For this review, take the finished solid that the model builds, in its own axes (mm). Face numbers are marked on the shaded views. A direction names the side the tool comes from. Give positions to 0.01 mm unless a question says otherwise; leave off trailing zeros. Order: outer loops, then holes, each group sorted by start corner. A loop starts at its lowest first (then second) coordinate and runs counter-clockwise, first axis right, second up.
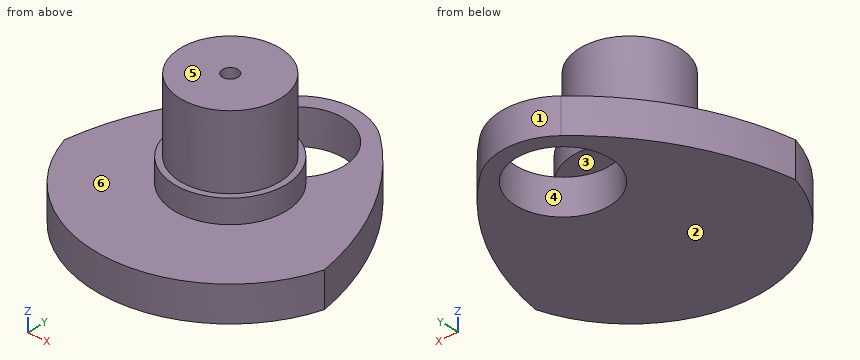
from build123d import *

# Parameters (mm, degrees)
SKETCH3_R           = 17
BOSS_EXTRUDE2_DEPTH = 25
SKETCH4_R           = 19
BOSS_EXTRUDE3_DEPTH = 8
BOSS_EXTRUDE4_DEPTH = 12
SKETCH9_R           = 16
CUT_EXTRUDE1_DEPTH  = 12
SKETCH10_R          = 2.65
CUT_EXTRUDE2_DEPTH  = 15


with BuildPart() as part:
    # Sketch3 → Boss-Extrude2 (new body)
    with BuildSketch(Plane.XY):
        Circle(SKETCH3_R)
    extrude(amount=BOSS_EXTRUDE2_DEPTH)

    # Sketch4 → Boss-Extrude3 (add)
    with BuildSketch(Plane.XY):
        Circle(SKETCH4_R)
    extrude(amount=-BOSS_EXTRUDE3_DEPTH)

    # Sketch5 → Boss-Extrude4 (add)
    with BuildSketch(Plane(origin=(0, 0, -8), x_dir=(-1, 0, 0), z_dir=(0, 0, -1))):
        with BuildLine():
            ThreePointArc((-44, -13.416407865), (0, -46), (44, -13.416407865))
            ThreePointArc((44, -13.416407865), (33.683444249, 16.469257624), (13.668094758, 40.943123461))
            ThreePointArc((13.668094758, 40.943123461), (0, 46), (-13.668094758, 40.943123461))
            ThreePointArc((-13.668094758, 40.943123461), (-33.683444249, 16.469257624), (-44, -13.416407865))
        make_face()
    extrude(amount=BOSS_EXTRUDE4_DEPTH)

    # Sketch9 → Cut-Extrude1 (cut)
    with BuildSketch(Plane(origin=(0, 0, -20), x_dir=(-1, 0, 0), z_dir=(0, 0, -1))):
        with Locations((0, 25)):
            Circle(SKETCH9_R)
    extrude(amount=-CUT_EXTRUDE1_DEPTH, mode=Mode.SUBTRACT)

    # Sketch10 → Cut-Extrude2 (cut)
    with BuildSketch(Plane.XY.offset(25)):
        Circle(SKETCH10_R)
    extrude(amount=-CUT_EXTRUDE2_DEPTH, mode=Mode.SUBTRACT)


solid = part.part
1) To check wall thickness, follow line 1 (Y direction, x = 0, z = 19); line 2 (Y direction, x = 0, z = -14); line 3 (Z direction, x = -33, y = -8). State the ranges of each line that lie inside material, in increasing order.
Answer sheet:
line 1: y = -17 to -2.65, 2.65 to 17
line 2: y = -46 to 9, 41 to 46
line 3: z = -20 to -8
2) We need section B-B on y = 25. Give the boundary of the cut face in (x, z), then the cut area to 3 significant figures.
Answer sheet:
outline: (-28.27, -20) - (-16, -20) - (-16, -8) - (-28.27, -8) - close; (16, -20) - (28.27, -20) - (28.27, -8) - (16, -8) - close
area: 295 mm2
3) Tool access review of the marked faces 5 and 6: name each direction out of +Z, -Z, +X, -X, +Y, -Y from which nothing blocks a thin tool from reaching the whole face with its end or side.
Answer sheet:
face 5: +Z, +X, -X, +Y, -Y
face 6: +Z
4) We need section A-A on x = 0. Give the boundary of the cut face in (y, z), then the cut area to 3 significant figures.
Answer sheet:
outline: (-46, -20) - (9, -20) - (9, -8) - (19, -8) - (19, 0) - (17, 0) - (17, 25) - (2.65, 25) - (2.65, 10) - (-2.65, 10) - (-2.65, 25) - (-17, 25) - (-17, 0) - (-19, 0) - (-19, -8) - (-46, -8) - close; (41, -20) - (46, -20) - (46, -8) - (41, -8) - close
area: 1,790 mm2
5) Clearance check with flat-ended pins moving along their axes: pin 1 (1.5 mm diameter, centred on y = -13, z = 12.5, fed in from +X); pin 2 (1 mm diameter, centred on x = -9.5, z = 5.5, fed in from -Y); pin 3 (8 mm diameter, centred on x = 32.5, y = -3, fed in from +Z); pin 4 (10 mm diameter, centred on y = 32, z = 1.5, fed in from -X). State where each tip first meets the part, or that it passes through.
Answer sheet:
pin 1: stops at x = 11.79
pin 2: stops at y = -14.42
pin 3: stops at z = -8
pin 4: passes through
6) Draft analysis for pull direction X (two halves, no side actions). For the marked faces 1, 2, 3 and 4, state which applies: +X half, -X half, draft (parallel to the pull), parting line (faces both ways), or undercut.
Answer sheet:
face 1: parting line
face 2: draft
face 3: undercut
face 4: undercut
7) We need section C-C on z = 19.5. Give the boundary of the cut face in (x, y), then the cut area to 3 significant figures.
Answer sheet:
outline: circle Ø34 at (0, 0); hole circle Ø5.3 at (0, 0)
area: 886 mm2
8) We need section D-D on y = -5.5. Give the boundary of the cut face in (x, z), then the cut area to 3 significant figures.
Answer sheet:
outline: (-42.39, -20) - (42.39, -20) - (42.39, -8) - (18.19, -8) - (18.19, 0) - (16.09, 0) - (16.09, 25) - (-16.09, 25) - (-16.09, 0) - (-18.19, 0) - (-18.19, -8) - (-42.39, -8) - close
area: 2,110 mm2
